Job drawing, mm, ordinate dimensions from the low corner. One solid piece. Coordinates: 2 decimals unless noted, no trailing zeros. Loops run counter-clockwise (first coordinate to the right, second up) from the corner with the lowest first, then second, coordinate; pieces in that order, holes last. Notation, with made-up numbers: (28, -5) - (85, -5) arc R19 cw to (85, 30) - close; hole circle Ø10 at (-26.75, 23). An arc over 180 degrees is marked (long way). Use a Markdown table: item, result. Add a question column.
1. Band-saw the part on B-B, the plane y = 3.85. Give the cut face in (x, z) (1 decimal), plus the area to 3 significant figures.
2. Band-saw the part on C-C, the plane z = 27.5. Count the separate pieces of the cut face and the enclosed holes in it, plus the area to 3 significant figures.
3. Drop flat-ended pins along their axis: pin 1 (1.5 mm diameter, centred on y = 1.5, z = 19.5, fed in from -X); pin 2 (3.5 mm diameter, centred on x = 6.24, z = 28.25, fed in from -Y); pin 3 (2 mm diameter, centred on y = 4, z = 23.5, fed in from -X); pin 4 (3 mm diameter, centred on x = 6.24, z = 7.75, fed in from +Y). Give the stop position or say it passes through.
4. Band-saw the part on A-A, the plane z = 18. Give the cut face in (x, y), plus the area to 3 significant figures.
5. Pull direction X, two halves, no side cores. Call the marked faces 1, 2 and 3: pulls with the +X half, pulls with the -X half, needs draft (parallel to the pull), parting line crosses it, or undercut.
6. Wall check: probe 1 along X at (y, z) = (3.2, 8.5); probe 2 along Z at (x, y) = (5.5, 3.3); probe 3 along Y at (x, z) = (15.5, 6). Give the ranges that are in metal, low to high. Write a range as [from, to].
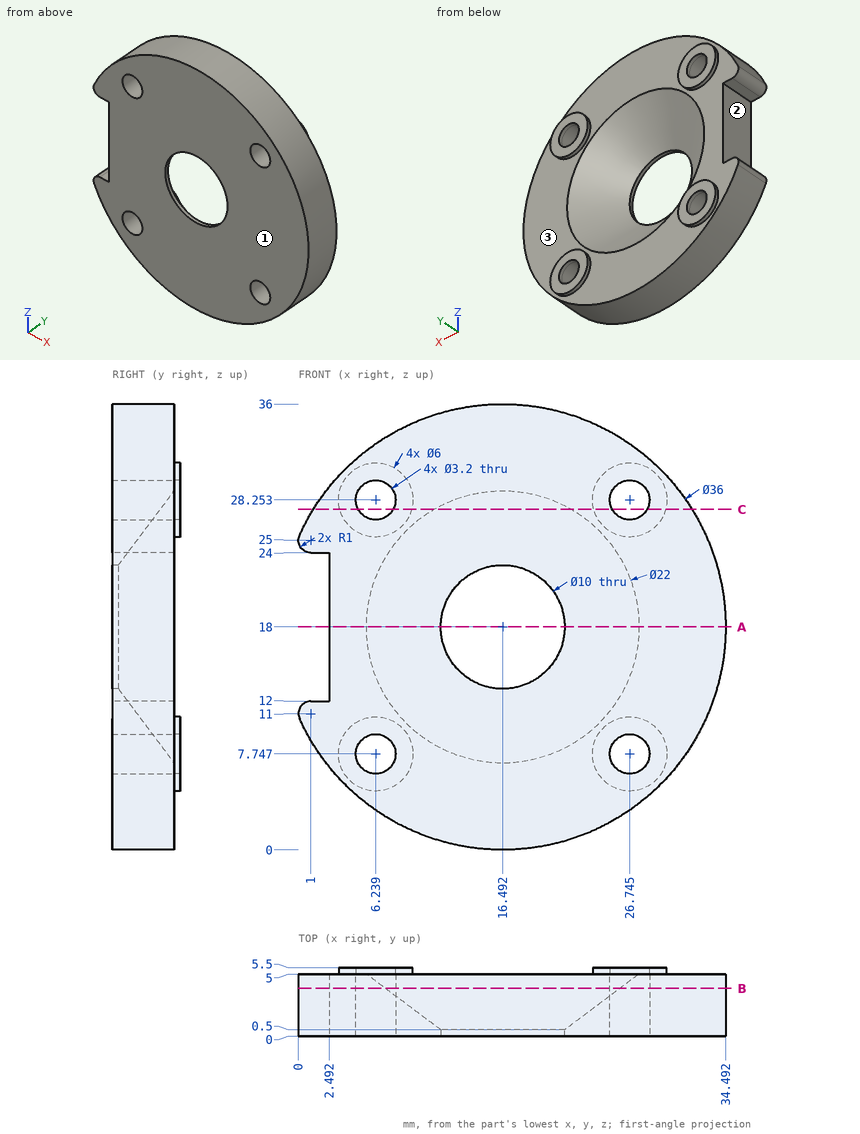
Geometry check:
| question | item | result |
|---|---|---|
| 1 | outline | (0.1, 10.6) arc R18 ccw (long way) to (0.1, 25.4) arc R1 ccw to (1, 24) - (2.5, 24) - (2.5, 12) - (1, 12) arc R1 ccw to start; hole circle Ø3.2 at (6.2, 7.7); hole circle Ø3.2 at (6.2, 28.3); hole circle Ø18.9 at (16.5, 18); hole circle Ø3.2 at (26.7, 7.7); hole circle Ø3.2 at (26.7, 28.3) |
| 1 | area | 659 mm^2 |
| 2 | separate pieces | 3 |
| 2 | enclosed holes | 0 |
| 2 | area | 119 mm^2 |
| 3 | pin 1 | stops at x = 2.49 |
| 3 | pin 2 | stops at y = 0 |
| 3 | pin 3 | stops at x = 0.13 |
| 3 | pin 4 | passes through |
| 4 | outline | (2.49, 0) - (11.49, 0) - (11.49, 0.5) - (5.49, 5) - (2.49, 5) - close; (21.49, 0) - (34.49, 0) - (34.49, 5) - (27.49, 5) - (21.49, 0.5) - close |
| 4 | area | 83.0 mm^2 |
| 5 | face 1 | needs draft |
| 5 | face 2 | pulls with the -X half |
| 5 | face 3 | undercut |
| 6 | probe 1 | x = [1.2, 4.83], [7.65, 25.33], [28.16, 31.78] |
| 6 | probe 2 | z = [3.75, 6.33], [9.17, 26.83], [29.67, 32.25] |
| 6 | probe 3 | y = [0, 5] |
